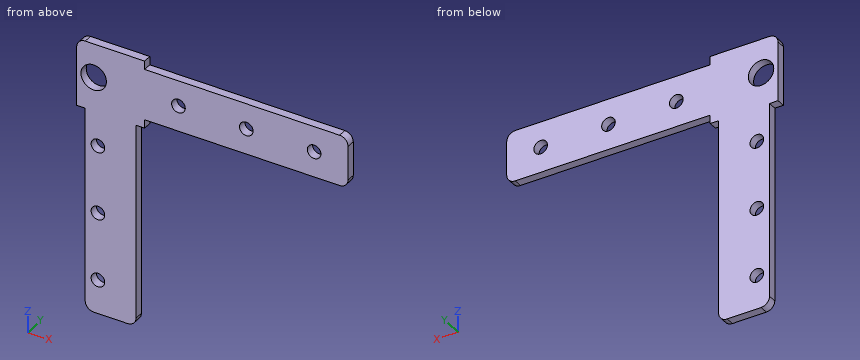
from build123d import *

# Parameters (mm, degrees)
BOSS_EXTRUDE1_DEPTH    = 3.175
F_10_CLEARANCE_HOLE1_D = 5.1054
SKETCH5_R              = 4.7625
CUT_EXTRUDE1_DEPTH     = 144.719172782
FILLET1_R              = 3.175


with BuildPart() as part:
    # Sketch2 → Boss-Extrude1 (new body)
    with BuildSketch(Plane(origin=(0, 0, 0), x_dir=(1, 0, 0), z_dir=(0, 1, 0))):
        Polygon((0, 0), (0, 25.4), (3.175, 25.4), (3.175, 101.6), (22.225, 101.6), (22.225, 25.4), (25.4, 25.4), (25.4, 22.225), (101.6, 22.225), (101.6, 3.175), (25.4, 3.175), (25.4, 0), align=None)
    extrude(amount=BOSS_EXTRUDE1_DEPTH)

    # #10 Clearance Hole1 (through all)
    with Locations(Plane(origin=(0, 3.175, 0), x_dir=(1, 0, 0), z_dir=(0, 1, 0))):
        with Locations((88.9, 12.7), (7.9375, 88.9), (7.9375, 63.5), (7.9375, 38.1), (38.1, 12.7), (63.5, 12.7)):
            Hole(F_10_CLEARANCE_HOLE1_D / 2)

    # Sketch5 → Cut-Extrude1 (cut, through all)
    with BuildSketch(Plane(origin=(0, 3.175, 0), x_dir=(1, 0, 0), z_dir=(0, 1, 0))):
        with Locations(Location((6.35, 12.7, 0), (0, 0, 270))):
            Circle(SKETCH5_R)
    extrude(amount=-CUT_EXTRUDE1_DEPTH, mode=Mode.SUBTRACT)

    # Fillet1
    fillet1_edges = [part.edges().sort_by_distance(p)[0] for p in [
        (0, 1.5875, 0),
        (3.175, 1.5875, -101.6),
        (22.225, 1.5875, -101.6),
        (101.6, 1.5875, -22.225),
        (101.6, 1.5875, -3.175),
    ]]
    fillet(fillet1_edges, radius=FILLET1_R)


solid = part.part
For this review, take the finished solid that the model builds, in its own axes (mm). Round coordinates to 2 decimals unless told otherwise and drop trailing zeros. Loops run counter-clockwise (first coordinate to the right, second up) from the corner with the lowest first, then second, coordinate; pieces in that order, holes last. Notation, with made-up numbers: (49.25, -13) - (99.25, -13) arc R24 ccw to (99.25, 4) - close; hole circle Ø8 at (69, 61). An arc over 180 degrees is marked (long way). Use one line per item in the form item = value.
1) We need section B-B on y = 0.5. State how many separate pieces and enclosed holes the cut face has, then the cut area to 3 significant figures.
Solutions:
separate_pieces = 1
enclosed_holes = 7
area = 3,340 mm2
2) We need section C-C on z = -12.7. Write out the cut boundary in (x, y) (1 decimal), then the cut area to 3 significant figures.
Solutions:
outline = (0, 0) - (1.6, 0) - (1.6, 3.2) - (0, 3.2) - close; (11.1, 0) - (35.5, 0) - (35.5, 3.2) - (11.1, 3.2) - close; (40.7, 0) - (60.9, 0) - (60.9, 3.2) - (40.7, 3.2) - close; (66.1, 0) - (86.3, 0) - (86.3, 3.2) - (66.1, 3.2) - close; (91.5, 0) - (101.6, 0) - (101.6, 3.2) - (91.5, 3.2) - close
area = 244 mm2
3) We need section A-A on x = 88.9. Write out the cut boundary in (y, z) (3 decimals), then the cut area to 3 significant figures.
Solutions:
outline = (0, -22.225) - (3.175, -22.225) - (3.175, -15.253) - (0, -15.253) - close; (0, -10.147) - (3.175, -10.147) - (3.175, -3.175) - (0, -3.175) - close
area = 44.3 mm2
4) Clearance check with flat-ended pins moving along their axes: P1, Ø1, axis at y = 1, z = -75.5, coming from the +X side (3 decimals); P2, Ø6, axis at x = 7.94, z = -88.9, coming from the +Y side (3 decimals); P3, Ø1.6, axis at x = 68, y = 1.5, coming from the -Z side (3 decimals); P4, Ø1.6, axis at y = 2, z = -1.5, coming from the +X side. State where each tip first meets the part, or that it passes through.
Solutions:
P1 = 22.225
P2 = 3.175
P3 = -22.225
P4 = 25.4
5) Wall thickness on probe 1 along X at (y, z) = (0.9, -12.7); probe 2 along Z at (x, y) = (63.5, 1.6) (3 decimals); probe 3 along X at (y, z) = (0.8, -88.9) (3 decimals): over which ranges is each line inside the solid? List them lowest first.
Solutions:
probe_1 = 0 to 1.59, 11.11 to 35.55, 40.65 to 60.95, 66.05 to 86.35, 91.45 to 101.6
probe_2 = -22.225 to -15.253, -10.147 to -3.175
probe_3 = 3.175 to 5.385, 10.49 to 22.225
6) We need section D-D on z = -63.5. Write out the cut boundary in (x, y) (3 decimals), then the cut area to 3 significant figures.
Solutions:
outline = (3.175, 0) - (5.385, 0) - (5.385, 3.175) - (3.175, 3.175) - close; (10.49, 0) - (22.225, 0) - (22.225, 3.175) - (10.49, 3.175) - close
area = 44.3 mm2
